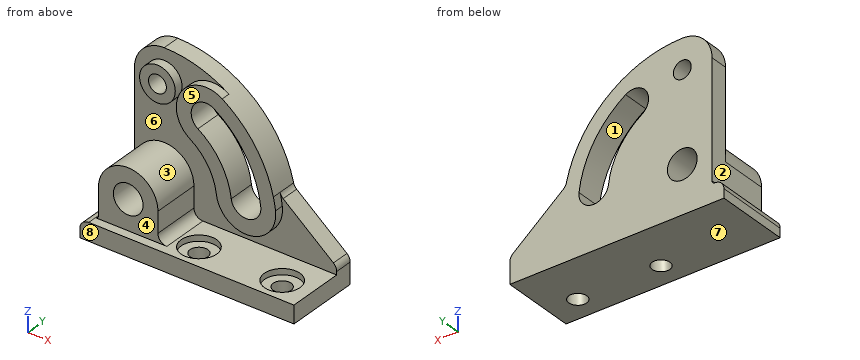
```python
from build123d import *

# Parameters (mm, degrees)
F1_DEPTH        = 25
F2_R            = 6
F3_DEPTH        = 19
F4_R            = 6
F5_DEPTH        = 16
F7_DEPTH        = 3
F9_D            = 10
F11_D           = 6
F13_DEPTH       = 9
F15_D           = 6
F15_CBORE_D     = 12
F15_CBORE_DEPTH = 2


with BuildPart() as f1:
    # F0 (on Front) → F1 (new body)
    with BuildSketch(Plane.XZ):
        with BuildLine():
            Line((-14, -16), (0, -16))
            Line((0, -16), (58, -16))
            Line((58, -16), (58, -8.9151388271))
            ThreePointArc((58, -8.9151388271), (57.7132792525, -7.6352498874), (56.9079228681, -6.6000080901))
            Line((56.9079228681, -6.6000080901), (39.9944124577, 7.3385884551))
            ThreePointArc((39.9944124577, 7.3385884551), (39.3510237496, 8.0754894114), (38.9789165822, 8.9802038996))
            ThreePointArc((38.9789165822, 8.9802038996), (24.9077482324, 31.2986274139), (0, 40))
            ThreePointArc((0, 40), (-7.0710678119, 37.0710678119), (-10, 30))
            Line((-10, 30), (-10, -9))
            ThreePointArc((-10, -9), (-10.2928932188, -9.7071067812), (-11, -10))
            ThreePointArc((-11, -10), (-13.1213203436, -10.8786796564), (-14, -13))
            Line((-14, -13), (-14, -16))
        make_face()
    extrude(amount=F1_DEPTH)

    # F2 (on face) → F3 (cut)
    with BuildSketch(Plane.XZ.offset(25)):
        with BuildLine():
            ThreePointArc((-10, 0), (0, 10), (10, 0))
            Line((10, 0), (10, -7))
            ThreePointArc((10, -7), (10.8786796564, -9.1213203436), (13, -10))
            Line((13, -10), (58, -10))
            Line((58, -10), (58, -8.9151388271))
            ThreePointArc((58, -8.9151388271), (57.7132792525, -7.6352498874), (56.9079228681, -6.6000080901))
            Line((56.9079228681, -6.6000080901), (39.9944124577, 7.3385884551))
            ThreePointArc((39.9944124577, 7.3385884551), (39.3510237496, 8.0754894114), (38.9789165822, 8.9802038996))
            ThreePointArc((38.9789165822, 8.9802038996), (39.3938985367, 6.9369127198), (39.7018460657, 4.8747737362))
            ThreePointArc((39.7018460657, 4.8747737362), (30.9950779833, -6.2693812143), (19.8509230328, 2.4373868681))
            ThreePointArc((19.8509230328, 2.4373868681), (16.9609619231, 10.5983852847), (10.8927807003, 16.7734113589))
            ThreePointArc((10.8927807003, 16.7734113589), (7.952465371, 30.6065073885), (21.7855614006, 33.5468227178))
            ThreePointArc((21.7855614006, 33.5468227178), (11.3606137882, 38.3527893947), (0, 40))
            ThreePointArc((0, 40), (-7.0710678119, 37.0710678119), (-10, 30))
            Line((-10, 30), (-10, 0))
        make_face()
        with Locations((0, 30)):
            Circle(F2_R, mode=Mode.SUBTRACT)
    extrude(amount=-F3_DEPTH, mode=Mode.SUBTRACT)

    # F4 (on face) → F5 (cut)
    with BuildSketch(Plane.XZ.offset(25)):
        with Locations((0, 30)):
            Circle(F4_R)
        with BuildLine():
            ThreePointArc((39.7018460657, 4.8747737362), (33.9219238463, 21.1967705693), (21.7855614006, 33.5468227178))
            ThreePointArc((21.7855614006, 33.5468227178), (7.952465371, 30.6065073885), (10.8927807003, 16.7734113589))
            ThreePointArc((10.8927807003, 16.7734113589), (16.9609619231, 10.5983852847), (19.8509230328, 2.4373868681))
            ThreePointArc((19.8509230328, 2.4373868681), (30.9950779833, -6.2693812143), (39.7018460657, 4.8747737362))
        make_face()
    extrude(amount=-F5_DEPTH, mode=Mode.SUBTRACT)

    # F6 (on face) → F7 (cut)
    with BuildSketch(Plane.XZ.offset(25)):
        with BuildLine():
            Line((-11, -10), (13, -10))
            ThreePointArc((13, -10), (10.8786796564, -9.1213203436), (10, -7))
            Line((10, -7), (10, 0))
            ThreePointArc((10, 0), (0, 10), (-10, 0))
            Line((-10, 0), (-10, -9))
            ThreePointArc((-10, -9), (-10.2928932188, -9.7071067812), (-11, -10))
        make_face()
    extrude(amount=-F7_DEPTH, mode=Mode.SUBTRACT)

    # F9 (through all)
    with Locations(Plane.XZ.offset(22)):
        with Locations((0, 0)):
            Hole(F9_D / 2)

    # F11 (through all)
    with Locations(Plane.XZ.offset(9)):
        with Locations((0, 30)):
            Hole(F11_D / 2)

    # F12 (on face) → F13 (cut)
    with BuildSketch(Plane.XZ.offset(9)):
        with BuildLine():
            ThreePointArc((34.7391153074, 4.2654270192), (29.6816833655, 18.5471742482), (19.0623662255, 29.3534698781))
            ThreePointArc((19.0623662255, 29.3534698781), (12.1458182107, 27.8833122134), (13.6159758754, 20.9667641986))
            ThreePointArc((13.6159758754, 20.9667641986), (21.2012024039, 13.2479816058), (24.813653791, 3.0467335851))
            ThreePointArc((24.813653791, 3.0467335851), (30.3857312663, -1.3066504561), (34.7391153074, 4.2654270192))
        make_face()
    extrude(amount=-F13_DEPTH, mode=Mode.SUBTRACT)

    # F15 (through all)
    with Locations(Plane.XY.offset(-10)):
        with Locations((20, -17), (48, -17)):
            CounterBoreHole(F15_D / 2, F15_CBORE_D / 2, F15_CBORE_DEPTH)


solid = f1.part
```
Design review of the part built by this model. Coordinates are the model's own, in mm. Face numbers are marked on the shaded views. A direction names the side the tool comes from. Give positions to 0.01 mm unless a question says otherwise; leave off trailing zeros. Order: outer loops, then holes, each group sorted by start corner. A loop starts at its lowest first (then second) coordinate and runs counter-clockwise, first axis right, second up. Notation, with made-up numbers: (79, -40) - (97, -40) arc R18 ccw to (97, -29) - close; hole circle Ø10 at (61, 23.25). An arc over 180 degrees is marked (long way). Use a Markdown table: item, result. Add a question column.
(1) Add section A-A on y = -17. Give the boundary of the cut face in (x, z).
(2) Add section C-C on x = 33. Give the boundary of the cut face in (y, z).
(3) Machinability: for the marked faces 1, 2, 3, 4 and 5, which of the approach directions +Z, -Z, +X, -X, +Y, -Y give a long, thin tool a straight path to every point of the face, cutting with its end or side? Answer none if there is none.
(4) Add section B-B on x = 2. Give the boundary of the cut face in (y, z), then the cut area to 3 significant figures.
(5) Mouldability with a two-part tool opening along Z and no side actions: class the marked faces 6, 7 and 8 as +Z half, -Z half, draft (parallel to the pull), parting line (faces both ways), or undercut.
(6) Wall thickness on probe 1 along X at (y, z) = (-21, -11); probe 2 along X at (y, z) = (-7, 27.5); probe 3 along Y at (x, z) = (20, -15): over which ranges is each line inside the solid? List them lowest first. Write a range as [from, to].
(7) Add section D-D on y = -2. Give the boundary of the cut face in (x, z).
(8) Clearance check with flat-ended pins moving along their axes: P1, Ø3, axis at y = -9.5, z = -6, coming from the -X side; P2, Ø25, axis at x = 33, z = 13.5, coming from the -Y side; P3, Ø4, axis at y = -10, z = -5, coming from the +X side. State where each tip first meets the part, or that it passes through.
Report:
| question | item | result |
|---|---|---|
| 1 | outline | (-14, -16) - (17, -16) - (17, -12) - (14, -12) - (14, -10) - (13, -10) arc R3 cw to (10, -7) - (10, 0) arc R10 ccw to (-10, 0) - (-10, -9) arc R1 cw to (-11, -10) arc R3 ccw to (-14, -13) - close; (23, -16) - (45, -16) - (45, -12) - (42, -12) - (42, -10) - (26, -10) - (26, -12) - (23, -12) - close; (51, -16) - (58, -16) - (58, -10) - (54, -10) - (54, -12) - (51, -12) - close; hole circle Ø10 at (0, 0) |
| 2 | outline | (-25, -16) - (0, -16) - (0, -0.17) - (-9, -0.17) - (-9, -5.81) - (-6, -5.81) - (-6, -10) - (-25, -10) - close; (-9, 11.66) - (0, 11.66) - (0, 22.61) - (-9, 22.61) - close |
| 3 | face 1 | +Y, -Y |
| 3 | face 2 | +Z, -X, +Y, -Y |
| 3 | face 3 | -Y |
| 3 | face 4 | +Z, +X, -X, -Y |
| 3 | face 5 | +Z, +X, -Y |
| 4 | outline | (-25, -16) - (0, -16) - (0, -4.58) - (-22, -4.58) - (-22, -10) - (-25, -10) - close; (-22, 4.58) - (0, 4.58) - (0, 27.76) - (-9, 27.76) - (-9, 24.34) - (-6, 24.34) - (-6, 9.8) - (-22, 9.8) - close; (-9, 32.24) - (0, 32.24) - (0, 39.95) - (-6, 39.95) - (-6, 35.66) - (-9, 35.66) - close |
| 4 | area | 559 mm² |
| 5 | face 6 | undercut |
| 5 | face 7 | -Z half |
| 5 | face 8 | draft |
| 6 | probe 1 | x = [-13.24, 15.53], [24.47, 43.53], [52.47, 58] |
| 6 | probe 2 | x = [-5.45, -1.66], [1.66, 5.45], [6.62, 11.92], [21.65, 29.05] |
| 6 | probe 3 | y = [-25, -20], [-14, 0] |
| 7 | outline | (-14, -16) - (58, -16) - (58, -8.92) arc R3 ccw to (56.91, -6.6) - (39.99, 7.34) arc R3 cw to (38.98, 8.98) arc R40 ccw to (0, 40) arc R10 ccw to (-10, 30) - (-10, -9) arc R1 cw to (-11, -10) arc R3 ccw to (-14, -13) - close; hole circle Ø10 at (0, 0); hole circle Ø6 at (0, 30); hole (13.62, 20.97) arc R25 cw to (24.81, 3.05) arc R5 ccw to (34.74, 4.27) arc R35 ccw to (19.06, 29.35) arc R5 ccw to start |
| 8 | P1 | stops at x = -10 |
| 8 | P2 | stops at y = -9 |
| 8 | P3 | stops at x = 36.99 |
